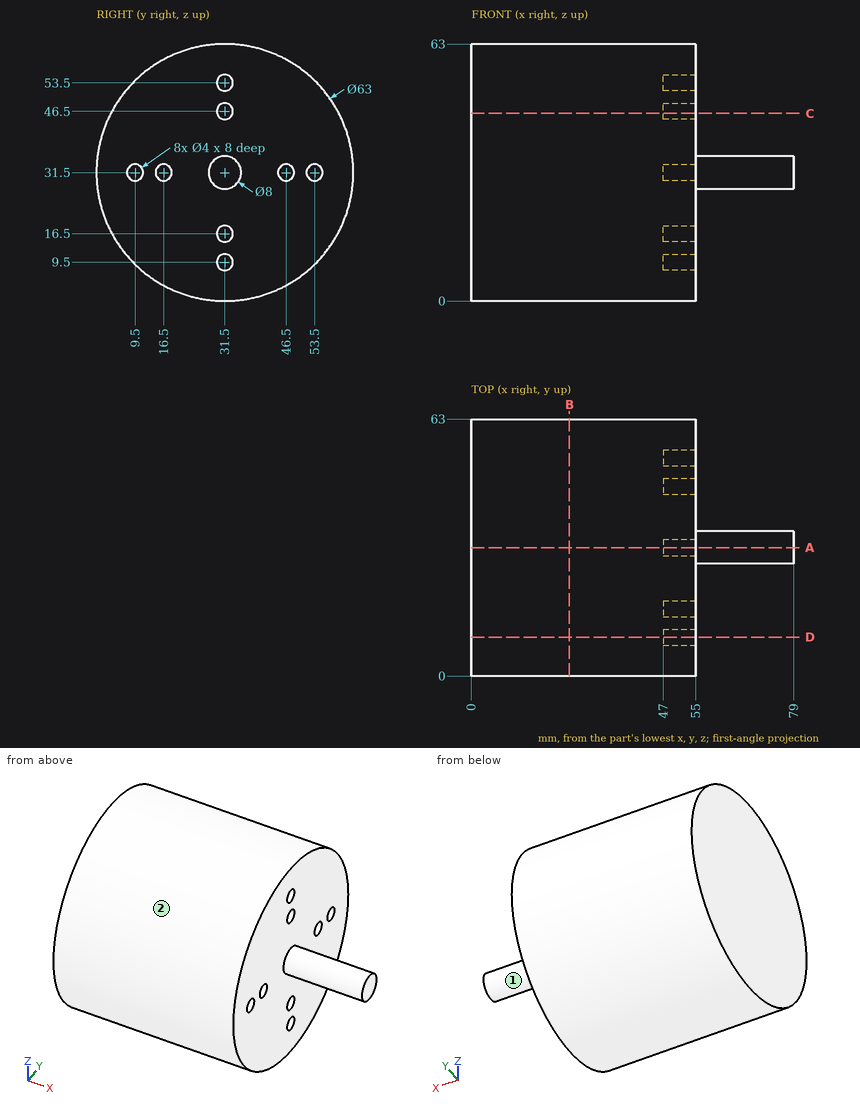
Here's the drawing with two shaded views (mm, measured from the low corner). I have some questions. A direction names the side the tool comes from. Round coordinates to 2 decimals unless told otherwise and drop trailing zeros. Order: outer loops, then holes, each group sorted by start corner. A loop starts at its lowest first (then second) coordinate and runs counter-clockwise, first axis right, second up. Notation, with made-up numbers: (-31, -3) -> (-8, -3) arc R23 ccw to (-8, 10) -> close; hole circle Ø7 at (6, 47.25). An arc over 180 degrees is marked (long way). Use a Markdown table: item, result. Add a question column.
(1) Suppose I cut it at D-D, the plane y = 9.5. Please give me the cut outline in (x, z).
(2) I need wall thicknesses on line 1 along X through (y, z) = (23.5, 49.5); line 2 along Z through (x, y) = (52, 33); line 3 along Z through (x, y) = (33.5, 32). Which ranges of each line are inside material? Lowest first, please.
(3) For pin 1 Ø3 at (y, z) = (31.5, 46.5) entering from -X; pin 2 Ø3 at (x, y) = (21.5, 49.5) entering from -Z; pin 3 Ø2 at (y, z) = (9, 32) entering from +X; pin 4 Ø4.5 at (y, z) = (17, 30.5) entering from +X, each with a flat end and sliding along its axis, tell me the tip position at first contact or that it passes through.
(4) For the marked faces 1 and 2, which set-ups out of +Z, -Z, +X, -X, +Y, -Y let a thin tool reach every point of the face, with its end or its side?
(5) Suppose I cut it at C-C, the plane z = 46. Please give me the cut outline in (x, y).
(6) Suppose I cut it at A-A, the plane y = 31.5. Please give me the cut outline in (x, z), and give its area (3 significant figures).
(7) Suppose I cut it at B-B, the plane x = 24. Please give me the cut outline in (y, z), and give its area (3 significant figures).
Verdict:
| question | item | result |
|---|---|---|
| 1 | outline | (0, 8.96) -> (55, 8.96) -> (55, 29.5) -> (47, 29.5) -> (47, 33.5) -> (55, 33.5) -> (55, 54.04) -> (0, 54.04) -> close |
| 2 | line 1 | 0 to 55 |
| 2 | line 2 | 0.04 to 8.18, 10.82 to 15.18, 17.82 to 45.18, 47.82 to 52.18, 54.82 to 62.96 |
| 2 | line 3 | 0 to 63 |
| 3 | pin 1 | x = 0 |
| 3 | pin 2 | z = 4.67 |
| 3 | pin 3 | x = 47 |
| 3 | pin 4 | x = 55 |
| 4 | face 1 | +X |
| 4 | face 2 | +X, -X |
| 5 | outline | (0, 3.54) -> (55, 3.54) -> (55, 29.56) -> (47, 29.56) -> (47, 33.44) -> (55, 33.44) -> (55, 59.46) -> (0, 59.46) -> close |
| 6 | outline | (0, 0) -> (55, 0) -> (55, 7.5) -> (47, 7.5) -> (47, 11.5) -> (55, 11.5) -> (55, 14.5) -> (47, 14.5) -> (47, 18.5) -> (55, 18.5) -> (55, 27.5) -> (79, 27.5) -> (79, 35.5) -> (55, 35.5) -> (55, 44.5) -> (47, 44.5) -> (47, 48.5) -> (55, 48.5) -> (55, 51.5) -> (47, 51.5) -> (47, 55.5) -> (55, 55.5) -> (55, 63) -> (0, 63) -> close |
| 6 | area | 3,530 mm2 |
| 7 | outline | circle Ø63 at (31.5, 31.5) |
| 7 | area | 3,120 mm2 |
